```python
from build123d import *

# Parameters (mm, degrees)
F0_W          = 114.3
F0_H          = 44.45
F1_DEPTH      = 127
F3_DEPTH      = 127
F7_DEPTH      = 139.954
F7_DEPTH_BACK = 86.614


with BuildPart() as f1:
    # F0 (on Right) → F1 (new body)
    with BuildSketch(Plane.YZ):
        with Locations((-12.579812, -6.85063)):
            Rectangle(F0_W, F0_H)
    extrude(amount=F1_DEPTH)

    # F2 (on Front) → F3 (cut, symmetric)
    with BuildSketch(Plane.XZ):
        Polygon((127, -29.07563), (127, 15.37437), (106.272625, 15.37437), align=None)
    extrude(amount=F3_DEPTH, both=True, mode=Mode.SUBTRACT)

    # F6 (on offset) → F7 (cut, two sides)
    with BuildSketch(Plane.YZ.offset(25.4)) as f7_sk:
        Polygon((-69.729812, 15.37437), (-69.729812, -29.07563), (-64.067963, 15.37437), align=None)
        Polygon((38.908338, 15.37437), (44.570188, -29.07563), (44.570188, 15.37437), align=None)
    extrude(amount=F7_DEPTH, mode=Mode.SUBTRACT)
    extrude(f7_sk.sketch, amount=-F7_DEPTH_BACK, mode=Mode.SUBTRACT)


solid = f1.part
```
Geometry check sheet. Reference: the model listing, model coordinates, mm. Coordinates: 2 decimals unless noted, no trailing zeros. Order: outer loops, then holes, each group sorted by start corner. A loop starts at its lowest first (then second) coordinate and runs counter-clockwise, first axis right, second up.
Q1. Thickness scan on probe 1 along X at (y, z) = (13.5, -13); probe 2 along Y at (x, z) = (37.5, -19.5); probe 3 along Y at (x, z) = (30, -0.5). Record the ranges inside material, lowest first.
Reply:
probe 1: x = 0 to 119.5
probe 2: y = -68.51 to 43.35
probe 3: y = -66.09 to 40.93
Q2. Sectioned sample at A-A on x = 14. Record the cut outline in (y, z).
Reply:
outline: (-69.73, -29.08) - (44.57, -29.08) - (38.91, 15.37) - (-64.07, 15.37) - close
Q3. Sectioned sample at B-B on y = 10. Record the cut outline in (x, z).
Reply:
outline: (0, -29.08) - (127, -29.08) - (106.27, 15.37) - (0, 15.37) - close
Q4. Depth check by flat-ended pin: pin 1 Ø2 at (x, z) = (94, 0) entering from -Y; pin 2 Ø12 at (y, z) = (13, -5.5) entering from +X; pin 3 Ø1 at (x, z) = (98, -22) entering from -Y. Enter the tip coordinate at first touch or a pass-through.
Reply:
pin 1: stops at y = -66.15
pin 2: stops at x = 118.8
pin 3: stops at y = -68.89
